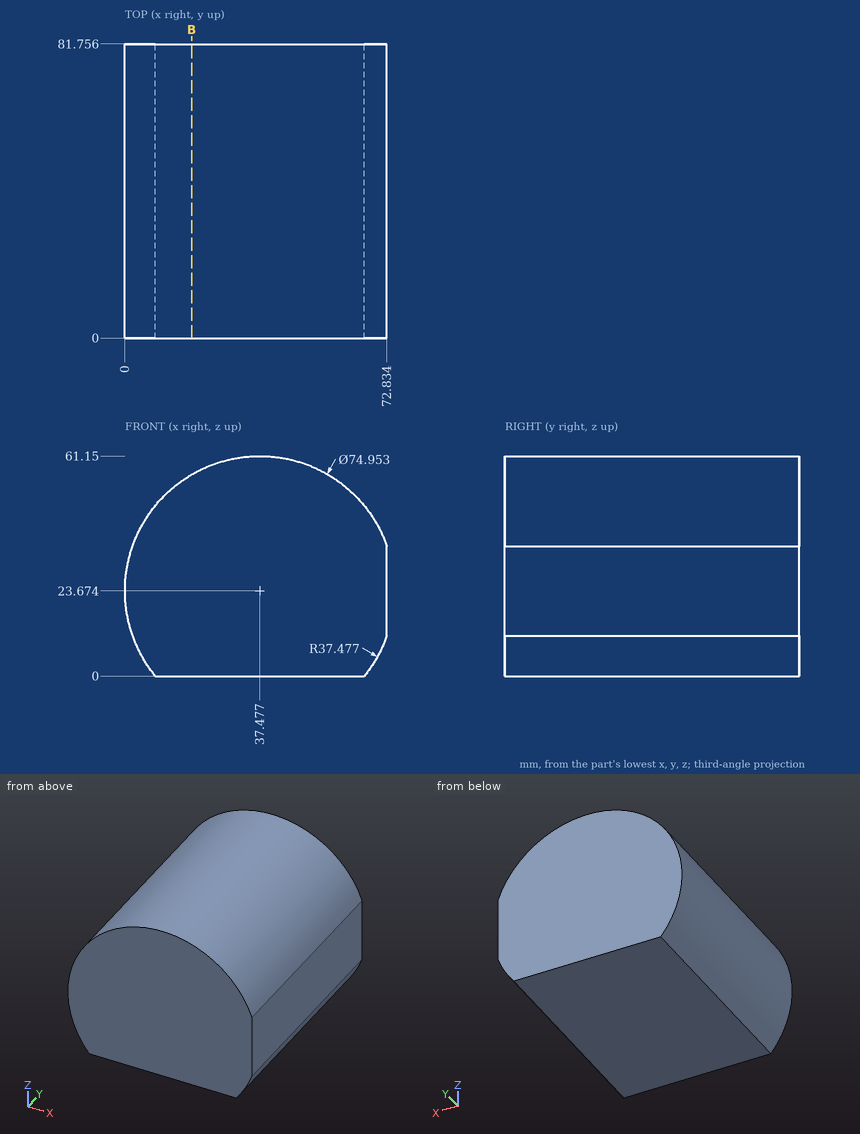
Design review of the part shown in the three views and the two pictorial views. Dimensions are in mm from the part's minimum x, y and z. Round coordinates to 2 decimals unless told otherwise and drop trailing zeros. Loops run counter-clockwise (first coordinate to the right, second up) from the corner with the lowest first, then second, coordinate; pieces in that order, holes last.
1) Wall thickness on line 1 along X through (y, z) = (66.5, 25); line 2 along X through (y, z) = (69.5, 47) (1 decimal); line 3 along Z through (x, y) = (39, 23.5): over which ranges is each line inside the solid? List them lowest first.
Values follow:
line 1: x = 0.02 to 72.83
line 2: x = 8.1 to 66.8
line 3: z = 0 to 61.12
2) Clearance check with flat-ended pins moving along their axes: P1, Ø1, axis at x = 33.5, y = 16.5, coming from the +Z side; P2, Ø5, axis at y = 35, z = 42, coming from the -X side (1 decimal); P3, Ø3, axis at y = 22, z = 51, coming from the +X side (1 decimal). State where each tip first meets the part, or that it passes through.
Values follow:
P1: stops at z = 60.99
P2: stops at x = 3.5
P3: stops at x = 64.6
3) Consider section B-B on x = 18.5. State the section outline as (y, z) points (1 decimal).
Values follow:
outline: (0, 0) - (81.8, 0) - (81.8, 56) - (0, 56) - close
